Geometry check sheet. Reference: the model listing, model coordinates, mm. Face numbers are marked on the shaded views. A direction names the side the tool comes from. Round coordinates to 2 decimals unless told otherwise and drop trailing zeros. Order: outer loops, then holes, each group sorted by start corner. A loop starts at its lowest first (then second) coordinate and runs counter-clockwise, first axis right, second up.
(1) Cross-section at C-C on z = -34. Enter the section's corners in (x, y), and give its area (3 significant figures).
(2) Thickness scan on L1, parallel to X at y = 24, z = -77; L2, parallel to X at y = 44, z = -111; L3, parallel to Z at x = -160.5, y = 15. Record the ranges inside material, lowest first.
(3) Cross-section at B-B on y = 23. Enter the section's corners in (x, z).
(4) Gauge pin test, flat ends, axial feed: P1, Ø4, axis at x = -127.5, z = -81.5, coming from the +Y side; P2, Ø1.5, axis at x = -180.5, z = -15, coming from the +Y side. Record the tip position at first contact, or that the pin passes through.
(5) Draft check along X on the marked faces 3, 4 and 5. Enter one of: pulls with the +X half, pulls with the -X half, needs draft (parallel to the pull), parting line crosses it, or undercut.
(6) Set-up check for the marked faces 1 and 2: record each of +Z, -Z, +X, -X, +Y, -Y from which the full face is reachable in a straight line by a thin tool's end or side.
(7) Cross-section at A-A on x = -122. Enter the section's corners in (y, z), and give its area (3 significant figures).
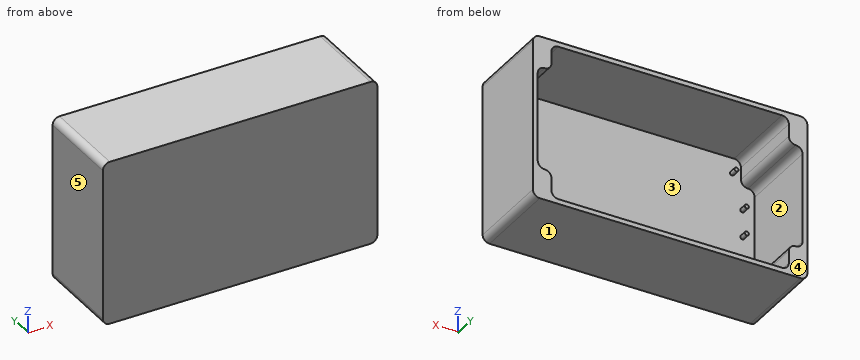
Autodesk Inventor part; units mm, degrees
ref_plane "YZ Plane" through (0, 0, 0) normal (1, 0, 0) x (0, 1, 0)
ref_plane "XZ Plane" through (0, 0, 0) normal (0, 1, 0) x (-1, 0, 0)
ref_plane "XY Plane" through (0, 0, 0) normal (0, 0, 1) x (1, 0, 0)
sketch "Sketch1" plane through (0, 0, 0) normal (0, 1, 0) x (-1, 0, 0)
  line L0 (0, 0) -> (200, 0)
  line L1 (200, 0) -> (200, -120)
  line L2 (200, -120) -> (0, -120)
  line L3 (0, -120) -> (0, 0)
  dimension "d0" = 200
  dimension "d1" = 120
extrude "Extrusion1" add sketch "Sketch1" along normal blind 3
sketch "Sketch2" plane through (0, 3, 0) normal (0, 1, 0) x (1, 0, 0)
  line L0 (-200, 0) -> (0, 0)
  line L1 (0, 0) -> (0, 120)
  line L2 (0, 120) -> (-200, 120)
  line L3 (-200, 120) -> (-200, 0)
  line L4 (-181.5, 116.5) -> (-18.5, 116.5)
  line L5 (-3.5, 92.5) -> (-3.5, 27.5)
  line L6 (-18.5, 3.5) -> (-181.5, 3.5)
  line L7 (-196.5, 27.5) -> (-196.5, 92.5)
  line L8 (-196.5, 3.5) -> (-186.5, 3.5)
  line L9 (-186.5, 8.5) -> (-186.5, 17.5)
  line L10 (-191.5, 22.5) -> (-191.5, 22.5)
  line L11 (-196.5, 22.5) -> (-196.5, 3.5)
  line L12 (-196.5, 116.5) -> (-186.5, 116.5)
  line L13 (-186.5, 111.5) -> (-186.5, 102.5)
  line L14 (-191.5, 97.5) -> (-191.5, 97.5)
  line L15 (-196.5, 97.5) -> (-196.5, 116.5)
  line L16 (-3.5, 116.5) -> (-13.5, 116.5)
  line L17 (-13.5, 111.5) -> (-13.5, 102.5)
  line L18 (-8.5, 97.5) -> (-8.5, 97.5)
  line L19 (-3.5, 97.5) -> (-3.5, 116.5)
  line L20 (-3.5, 3.5) -> (-13.5, 3.5)
  line L21 (-13.5, 8.5) -> (-13.5, 17.5)
  line L22 (-8.5, 22.5) -> (-8.5, 22.5)
  line L23 (-3.5, 22.5) -> (-3.5, 3.5)
  arc A0 (-3.5, 92.5) -> (-8.5, 97.5) centre (-8.5, 92.5) ccw
  arc A1 (-13.5, 111.5) -> (-18.5, 116.5) centre (-18.5, 111.5) ccw
  arc A2 (-8.5, 22.5) -> (-3.5, 27.5) centre (-8.5, 27.5) ccw
  arc A3 (-18.5, 3.5) -> (-13.5, 8.5) centre (-18.5, 8.5) ccw
  arc A4 (-186.5, 8.5) -> (-181.5, 3.5) centre (-181.5, 8.5) ccw
  arc A5 (-196.5, 27.5) -> (-191.5, 22.5) centre (-191.5, 27.5) ccw
  arc A6 (-191.5, 97.5) -> (-196.5, 92.5) centre (-191.5, 92.5) ccw
  arc A7 (-181.5, 116.5) -> (-186.5, 111.5) centre (-181.5, 111.5) ccw
  arc A8 (-191.5, 97.5) -> (-186.5, 102.5) centre (-191.5, 102.5) ccw
  arc A9 (-186.5, 17.5) -> (-191.5, 22.5) centre (-191.5, 17.5) ccw
  arc A10 (-8.5, 22.5) -> (-13.5, 17.5) centre (-8.5, 17.5) ccw
  arc A11 (-13.5, 102.5) -> (-8.5, 97.5) centre (-8.5, 102.5) ccw
  line L24 (-196.5, 116.5) -> (-200, 116.5)
  line L25 (-196.5, 3.5) -> (-200, 3.5)
  line L26 (-3.5, 3.5) -> (-3.5, 0)
  line L27 (-3.5, 116.5) -> (-3.5, 120)
  line L28 (-196.5, 3.5) -> (-196.5, 0)
  point P0 (-186.5, 22.5)
  point P1 (-186.5, 97.5)
  point P2 (-13.5, 97.5)
  point P3 (-13.5, 22.5)
  dimension "d4" = 3.5
  dimension "d7" = 10
  dimension "d8" = 19
  dimension "d9" = 10
  dimension "d10" = 19
  dimension "d11" = 10
  dimension "d12" = 19
  dimension "d13" = 10
  dimension "d14" = 19
  dimension "d15" = 5
  dimension "d16" = 5
  dimension "d17" = 5
  dimension "d18" = 5
  dimension "d19" = 5
  dimension "d20" = 5
  dimension "d21" = 5
  dimension "d22" = 5
  dimension "d23" = 5
  dimension "d73" = 3.5
  dimension "d74" = 3.5
  dimension "d75" = 3.5
  dimension "d78" = 3.5
extrude "Extrusion2" add sketch "Sketch2" along normal blind 60
sketch "Sketch3" plane through (0, 3, 0) normal (0, 1, 0) x (1, 0, 0)
  line L0 (-200, 120) -> (-200, 105)
  line L1 (-200, 120) -> (-200, 0)
  line L2 (0, 120) -> (0, 0)
  line L3 (0, 0) -> (0, 15)
  line L4 (-181.5, 3.5) -> (-18.5, 3.5)
  circle A0 centre (-180, 105) radius 1.5
  line L5 (-180, 105) -> (-158, 105)
  circle A1 centre (-158, 105) radius 1.5
  circle A2 centre (-187.5, 60) radius 1.5
  line L6 (-187.5, 60) -> (-187.5, 80)
  line L7 (-187.5, 60) -> (-187.5, 40)
  circle A3 centre (-187.5, 40) radius 1.5
  circle A4 centre (-187.5, 80) radius 1.5
  line L8 (-200, 0) -> (-200, 120)
  line L9 (-187.5, 60) -> (-12.5, 60)
  circle A5 centre (-12.5, 60) radius 1.5
  line L10 (0, 120) -> (-200, 120)
  line L11 (-100, 120) -> (-100, 0)
  line L12 (0, 0) -> (-200, 0)
  circle A6 centre (-20, 105) radius 1.5
  line L13 (-180, 105) -> (-181.5, 105)
  line L14 (-184, 106) -> (-200, 106)
  line L15 (-180, 105) -> (-159.5, 105)
  line L16 (-180, 15) -> (-20, 15)
  circle A7 centre (-180, 15) radius 1.5
  line L17 (-84.857, 105) -> (-84.857, 15)
  line L18 (-158, 105) -> (-20, 105)
  circle A8 centre (-20, 15) radius 1.5
  line L19 (-12.5, 60) -> (-12.5, 40)
  line L20 (-12.5, 60) -> (-12.5, 80)
  circle A9 centre (-12.5, 80) radius 1.5
  circle A10 centre (-12.5, 40) radius 1.5
  line L21 (-180, 105) -> (-20, 105)
  line L22 (-13.5, 111.5) -> (-13.5, 102.5)
  point P0 (-100, 60)
  point P1 (-100, 15)
  point P2 (-84.857, 60)
  point P3 (-100, 105)
  dimension "d35" = 3
  dimension "d37" = 3
  dimension "d24" = 15
  dimension "d36" = 22
  dimension "d41" = 3
  dimension "d44" = 20
  dimension "d45" = 20
  dimension "d54" = 175
  dimension "d55" = 3
  dimension "d57" = 3
  dimension "d59" = 160
  dimension "d60" = 3
  dimension "d62" = 90
  dimension "d63" = 3
  dimension "d64" = 20
  dimension "d65" = 20
  dimension "d66" = 3
  dimension "d67" = 3
  dimension "d68" = 3
  dimension "d69" = 3
  dimension "d72" = 138
fillet "Fillet2" radius 5 4 edges at (0, 31.5, 0) (0, 31.5, -120) (-200, 31.5, -120) (-200, 31.5, 0)
extrude "Extrusion4" add sketch "Sketch3" along normal blind 5.6 contours A7 | A3 | A4 | A2 L7 L9 | L9 L6 A2 | A0 L13 L5 | L5 L13 A0 | A1 L5 L18 | L18 L5 A1 | A6 | A9 | A10 | A5 L20 L9 | L9 L19 A5 | A8 | L6 L7 A2 | L20 A5 L19
properties part number "boks"
Found:
1. outline: (-200, 0) - (0, 0) - (0, 63) - (-3.5, 63) - (-3.5, 3) - (-196.5, 3) - (-196.5, 63) - (-200, 63) - close
1. area: 1,020 mm2
2. L1: x = -200 to -196.5, -3.5 to 0
2. L2: x = -200 to -186.5, -13.5 to 0
2. L3: z = -120 to -116.5, -3.5 to 0
3. outline: (-200, -115) arc R5 ccw to (-195, -120) - (-5, -120) arc R5 ccw to (0, -115) - (0, -5) arc R5 ccw to (-5, 0) - (-195, 0) arc R5 ccw to (-200, -5) - close; hole (-196.5, -92.5) arc R5 ccw to (-191.5, -97.5) arc R5 cw to (-186.5, -102.5) - (-186.5, -111.5) arc R5 ccw to (-181.5, -116.5) - (-18.5, -116.5) arc R5 ccw to (-13.5, -111.5) - (-13.5, -102.5) arc R5 cw to (-8.5, -97.5) arc R5 ccw to (-3.5, -92.5) - (-3.5, -27.5) arc R5 ccw to (-8.5, -22.5) arc R5 cw to (-13.5, -17.5) - (-13.5, -8.5) arc R5 ccw to (-18.5, -3.5) - (-181.5, -3.5) arc R5 ccw to (-186.5, -8.5) - (-186.5, -17.5) arc R5 cw to (-191.5, -22.5) arc R5 ccw to (-196.5, -27.5) - close
4. P1: stops at y = 3
4. P2: stops at y = 8.6
5. face 3: undercut
5. face 4: needs draft
5. face 5: pulls with the -X half
6. face 1: -Z, +X, -X, +Y, -Y
6. face 2: +Y
7. outline: (0, -120) - (63, -120) - (63, -116.5) - (3, -116.5) - (3, -3.5) - (63, -3.5) - (63, 0) - (0, 0) - close
7. area: 780 mm2
